Check sheet for the modelled part. Datum: model origin and axes. Units: mm. A direction names the side the tool comes from. Round coordinates to 2 decimals unless told otherwise and drop trailing zeros. Loops run counter-clockwise (first coordinate to the right, second up) from the corner with the lowest first, then second, coordinate; pieces in that order, holes last. Notation, with made-up numbers: (-2.75, 25) -> (14.25, 25) arc R21 cw to (14.25, 41) -> close; hole circle Ø10 at (-2.5, 44). An arc over 180 degrees is marked (long way). One line per item, written item: value. Start each with the question number.
1. Cross-section at B-B on y = 6.25. Record the cut outline in (x, z), then the cut area to 3 significant figures.
2. Set-up check for faces 1 (the face through (1, 22, 0)), 2 (the face through (-1, 22, 0)), 3 (the face through (0, 0, 0)): record each of +Z, -Z, +X, -X, +Y, -Y from which the full face is reachable in a straight line by a thin tool's end or side.
3. Material ranges on L1, parallel to Y at x = 0.95, z = 0.5; L2, parallel to X at y = 6.5, z = -0.2; L3, parallel to Z at x = -0.1, y = 20.75, recorded low to high.
4. Cross-section at D-D on z = -1. Record the cut outline in (x, y), then the cut area to 3 significant figures.
5. Cross-section at A-A on z = 0.55. Record the cut outline in (x, y).
6. Cross-section at C-C on x = -0.8. Record the cut outline in (y, z), then the cut area to 3 significant figures.
from build123d import *

# Parameters (mm, degrees)
SKETCH2_R               = 1.75
BOSS_EXTRUDE2_DEPTH     = 28
CUT_EXTRUDE1_START      = -6
CUT_EXTRUDE1_DEPTH      = 6
CUT_EXTRUDE2_DEPTH      = 29.263177076
CUT_EXTRUDE2_DEPTH_BACK = 29.263177076


with BuildPart() as part:
    # Sketch2 → Boss-Extrude2 (new body)
    with BuildSketch(Plane(origin=(0, 0, 0), x_dir=(1, 0, 0), z_dir=(0, 1, 0))):
        with Locations(Location((0, 0, 0), (0, 0, 270))):
            Circle(SKETCH2_R)
    extrude(amount=BOSS_EXTRUDE2_DEPTH)

    # Sketch5 → Cut-Extrude1 (cut)
    with BuildSketch(Plane(origin=(0, 28, 0), x_dir=(1, 0, 0), z_dir=(0, 1, 0)).offset(CUT_EXTRUDE1_START)):
        with BuildLine():
            Line((0.5, 1.677050983), (0.5, -1.677050983))
            ThreePointArc((0.5, -1.677050983), (1.75, 0), (0.5, 1.677050983))
        make_face()
        with BuildLine():
            Line((-0.5, -1.677050983), (-0.5, 1.677050983))
            ThreePointArc((-0.5, 1.677050983), (-1.75, 0), (-0.5, -1.677050983))
        make_face()
    extrude(amount=CUT_EXTRUDE1_DEPTH, mode=Mode.SUBTRACT)

    # Sketch9 → Cut-Extrude2 (cut, two sides: drawn at the far end of the back side and taken through both)
    with BuildSketch(Plane(origin=(0, 0, 1.677050983), x_dir=(-1, 0, 0), z_dir=(0, 0, -1)).offset(-CUT_EXTRUDE2_DEPTH_BACK)):
        Polygon((0.5, 22), (0.5, 28), (0.185553324, 28), align=None)
        Polygon((-0.5, 22), (-0.5, 28), (-0.185553324, 28), align=None)
    extrude(amount=CUT_EXTRUDE2_DEPTH + CUT_EXTRUDE2_DEPTH_BACK, mode=Mode.SUBTRACT)


solid = part.part
Taken from the geometry:
1. outline: circle Ø3.5 at (0, 0)
1. area: 9.62 mm2
2. face 1: +Z, -Z, +X, +Y
2. face 2: +Z, -Z, -X, +Y
2. face 3: +Z, -Z, +X, -X, -Y
3. L1: y = 0 to 22
3. L2: x = -1.74 to 1.74
3. L3: z = -1.75 to 1.75
4. outline: (-1.44, 0) -> (1.44, 0) -> (1.44, 22) -> (0.5, 22) -> (0.19, 28) -> (-0.19, 28) -> (-0.5, 22) -> (-1.44, 22) -> close
4. area: 67.3 mm2
5. outline: (-1.66, 0) -> (1.66, 0) -> (1.66, 22) -> (0.5, 22) -> (0.19, 28) -> (-0.19, 28) -> (-0.5, 22) -> (-1.66, 22) -> close
6. outline: (0, -1.56) -> (22, -1.56) -> (22, 1.56) -> (0, 1.56) -> close
6. area: 68.5 mm2
